Can you work these out from the model? Positions are in its coordinate system, mm. A direction names the side the tool comes from. Coordinates: 2 decimals unless noted, no trailing zeros. Order: outer loops, then holes, each group sorted by start corner. A loop starts at its lowest first (then second) coordinate and runs counter-clockwise, first axis right, second up. Notation, with made-up numbers: (-2.75, 68) -> (4.25, 68) arc R23 ccw to (4.25, 97) -> close; hole circle Ø5 at (26.25, -36.5). An arc over 180 degrees is marked (long way). Answer as CSV lines item,"result".
from build123d import *

# Parameters (mm, degrees)
SALIENTE_EXTRUIR1_DEPTH           = 10.5
CORTAR_EXTRUIR2_REACH             = 29.665
CROQUIS1_6_R                      = 1.15
CORTAR_EXTRUIR2_DIRECTION_2_REACH = 29.665
VACIADO3_T                        = -1
VACIADO3_THICKNESS_2_DEPTH        = 1
SALIENTE_EXTRUIR2_START           = 10.5
SALIENTE_EXTRUIR2_DEPTH           = 0.5
CROQUIS4_R                        = 1.15
CORTAR_EXTRUIR3_DEPTH             = 1
CROQUIS5_W                        = 6.4
CROQUIS5_H                        = 3.4
CORTAR_EXTRUIR4_DEPTH             = 0.8
CHAFL_N2_SIZE                     = 0.5
SALIENTE_EXTRUIR3_START           = -0.8
CROQUIS5_3_W                      = 6.2
CROQUIS5_3_H                      = 3.2
CROQUIS5_3_W_2                    = 5.6
CROQUIS5_3_H_2                    = 2.6
SALIENTE_EXTRUIR3_DEPTH           = 1.5
CROQUIS5_4_W                      = 5.4
CROQUIS5_4_H                      = 7.9
CORTAR_EXTRUIR5_DEPTH             = 35.965840473
SALIENTE_EXTRUIR4_START           = -0.8
CROQUIS5_6_R                      = 0.3
SALIENTE_EXTRUIR4_DEPTH           = 1.4
CROQUIS5_7_W                      = 1.3
CROQUIS5_7_H                      = 21
SALIENTE_EXTRUIR5_DEPTH           = 0.6


with BuildPart() as part:
    # Croquis1 → Saliente-Extruir1 (new, symmetric)
    with BuildSketch(Plane(origin=(0, 0, 0), x_dir=(1, 0, 0), z_dir=(0, 1, 0))):
        with BuildLine():
            Line((-9.7, 22.5), (9.7, 22.5))
            ThreePointArc((9.7, 22.5), (11.467766953, 21.767766953), (12.2, 20))
            Line((12.2, 20), (12.2, -20))
            ThreePointArc((12.2, -20), (11.467766953, -21.767766953), (9.7, -22.5))
            Line((9.7, -22.5), (-9.7, -22.5))
            ThreePointArc((-9.7, -22.5), (-11.467766953, -21.767766953), (-12.2, -20))
            Line((-12.2, -20), (-12.2, 20))
            ThreePointArc((-12.2, 20), (-11.467766953, 21.767766953), (-9.7, 22.5))
        make_face()
    extrude(amount=SALIENTE_EXTRUIR1_DEPTH, both=True)

    # Croquis1<6> → Cortar-Extruir2 (cut, up to next)
    with BuildSketch(Plane(origin=(0, 0, 0), x_dir=(1, 0, 0), z_dir=(0, 1, 0)), mode=Mode.PRIVATE) as cortar_extruir2_sk1:
        with Locations(Location((-9.93, 20.23, 0), (0, 0, 270))):
            Circle(CROQUIS1_6_R)
    cortar_extruir2_tool1 = extrude(cortar_extruir2_sk1.sketch, amount=-CORTAR_EXTRUIR2_REACH, mode=Mode.PRIVATE) & part.part
    # Croquis1<6> → Cortar-Extruir2 (cut, up to next)
    with BuildSketch(Plane(origin=(0, 0, 0), x_dir=(1, 0, 0), z_dir=(0, 1, 0)), mode=Mode.PRIVATE) as cortar_extruir2_sk2:
        with Locations(Location((9.93, 20.23, 0), (0, 0, 270))):
            Circle(CROQUIS1_6_R)
    cortar_extruir2_tool2 = extrude(cortar_extruir2_sk2.sketch, amount=-CORTAR_EXTRUIR2_REACH, mode=Mode.PRIVATE) & part.part
    # Croquis1<6> → Cortar-Extruir2 (cut, up to next)
    with BuildSketch(Plane(origin=(0, 0, 0), x_dir=(1, 0, 0), z_dir=(0, 1, 0)), mode=Mode.PRIVATE) as cortar_extruir2_sk3:
        with Locations(Location((-9.93, -20.23, 0), (0, 0, 270))):
            Circle(CROQUIS1_6_R)
    cortar_extruir2_tool3 = extrude(cortar_extruir2_sk3.sketch, amount=-CORTAR_EXTRUIR2_REACH, mode=Mode.PRIVATE) & part.part
    # Croquis1<6> → Cortar-Extruir2 (cut, up to next)
    with BuildSketch(Plane(origin=(0, 0, 0), x_dir=(1, 0, 0), z_dir=(0, 1, 0)), mode=Mode.PRIVATE) as cortar_extruir2_sk4:
        with Locations(Location((9.93, -20.23, 0), (0, 0, 270))):
            Circle(CROQUIS1_6_R)
    cortar_extruir2_tool4 = extrude(cortar_extruir2_sk4.sketch, amount=-CORTAR_EXTRUIR2_REACH, mode=Mode.PRIVATE) & part.part
    add(cortar_extruir2_tool1.solids().sort_by_distance((-9.93, 0, -20.23))[0], mode=Mode.SUBTRACT)
    add(cortar_extruir2_tool2.solids().sort_by_distance((9.93, 0, -20.23))[0], mode=Mode.SUBTRACT)
    add(cortar_extruir2_tool3.solids().sort_by_distance((-9.93, 0, 20.23))[0], mode=Mode.SUBTRACT)
    add(cortar_extruir2_tool4.solids().sort_by_distance((9.93, 0, 20.23))[0], mode=Mode.SUBTRACT)

    # Croquis1<6> → Cortar-Extruir2 direction 2 (cut, up to next)
    with BuildSketch(Plane(origin=(0, 0, 0), x_dir=(1, 0, 0), z_dir=(0, 1, 0)), mode=Mode.PRIVATE) as cortar_extruir2_direction_2_sk1:
        with Locations(Location((-9.93, 20.23, 0), (0, 0, 270))):
            Circle(CROQUIS1_6_R)
    cortar_extruir2_direction_2_tool1 = extrude(cortar_extruir2_direction_2_sk1.sketch, amount=CORTAR_EXTRUIR2_DIRECTION_2_REACH, mode=Mode.PRIVATE) & part.part
    # Croquis1<6> → Cortar-Extruir2 direction 2 (cut, up to next)
    with BuildSketch(Plane(origin=(0, 0, 0), x_dir=(1, 0, 0), z_dir=(0, 1, 0)), mode=Mode.PRIVATE) as cortar_extruir2_direction_2_sk2:
        with Locations(Location((9.93, 20.23, 0), (0, 0, 270))):
            Circle(CROQUIS1_6_R)
    cortar_extruir2_direction_2_tool2 = extrude(cortar_extruir2_direction_2_sk2.sketch, amount=CORTAR_EXTRUIR2_DIRECTION_2_REACH, mode=Mode.PRIVATE) & part.part
    # Croquis1<6> → Cortar-Extruir2 direction 2 (cut, up to next)
    with BuildSketch(Plane(origin=(0, 0, 0), x_dir=(1, 0, 0), z_dir=(0, 1, 0)), mode=Mode.PRIVATE) as cortar_extruir2_direction_2_sk3:
        with Locations(Location((-9.93, -20.23, 0), (0, 0, 270))):
            Circle(CROQUIS1_6_R)
    cortar_extruir2_direction_2_tool3 = extrude(cortar_extruir2_direction_2_sk3.sketch, amount=CORTAR_EXTRUIR2_DIRECTION_2_REACH, mode=Mode.PRIVATE) & part.part
    # Croquis1<6> → Cortar-Extruir2 direction 2 (cut, up to next)
    with BuildSketch(Plane(origin=(0, 0, 0), x_dir=(1, 0, 0), z_dir=(0, 1, 0)), mode=Mode.PRIVATE) as cortar_extruir2_direction_2_sk4:
        with Locations(Location((9.93, -20.23, 0), (0, 0, 270))):
            Circle(CROQUIS1_6_R)
    cortar_extruir2_direction_2_tool4 = extrude(cortar_extruir2_direction_2_sk4.sketch, amount=CORTAR_EXTRUIR2_DIRECTION_2_REACH, mode=Mode.PRIVATE) & part.part
    add(cortar_extruir2_direction_2_tool1.solids().sort_by_distance((-9.93, 0, -20.23))[0], mode=Mode.SUBTRACT)
    add(cortar_extruir2_direction_2_tool2.solids().sort_by_distance((9.93, 0, -20.23))[0], mode=Mode.SUBTRACT)
    add(cortar_extruir2_direction_2_tool3.solids().sort_by_distance((-9.93, 0, 20.23))[0], mode=Mode.SUBTRACT)
    add(cortar_extruir2_direction_2_tool4.solids().sort_by_distance((9.93, 0, 20.23))[0], mode=Mode.SUBTRACT)

    # Vaciado3
    vaciado3_openings = [part.faces().sort_by_distance(p)[0] for p in [
        (0, -10.5, 0),
    ]]
    offset(amount=VACIADO3_T, openings=vaciado3_openings, kind=Kind.INTERSECTION)

    # Vaciado3 thickness 2 face (on inner face of the shell) → Vaciado3 thickness 2 (add)
    with BuildSketch(Plane.ZX.offset(9.5)):
        with BuildLine():
            Line((-21.5, -8.195180125), (-21.5, 8.195180125))
            ThreePointArc((-21.5, 8.195180125), (-18.70972042, 8.40972042), (-18.495180125, 11.2))
            Line((-18.495180125, 11.2), (18.495180125, 11.2))
            ThreePointArc((18.495180125, 11.2), (18.70972042, 8.40972042), (21.5, 8.195180125))
            Line((21.5, 8.195180125), (21.5, -8.195180125))
            ThreePointArc((21.5, -8.195180125), (18.70972042, -8.40972042), (18.495180125, -11.2))
            Line((18.495180125, -11.2), (-18.495180125, -11.2))
            ThreePointArc((-18.495180125, -11.2), (-18.70972042, -8.40972042), (-21.5, -8.195180125))
        make_face()
    extrude(amount=-VACIADO3_THICKNESS_2_DEPTH)

    # Croquis1<4> → Saliente-Extruir2 (add)
    with BuildSketch(Plane(origin=(0, 0, 0), x_dir=(1, 0, 0), z_dir=(0, 1, 0)).offset(SALIENTE_EXTRUIR2_START)):
        with BuildLine():
            ThreePointArc((9.7, 22), (11.114213562, 21.414213562), (11.7, 20))
            Line((11.7, 20), (11.7, -20))
            ThreePointArc((11.7, -20), (11.114213562, -21.414213562), (9.7, -22))
            Line((9.7, -22), (-9.7, -22))
            ThreePointArc((-9.7, -22), (-11.114213562, -21.414213562), (-11.7, -20))
            Line((-11.7, -20), (-11.7, 20))
            ThreePointArc((-11.7, 20), (-11.114213562, 21.414213562), (-9.7, 22))
            Line((-9.7, 22), (9.7, 22))
        make_face()
        with BuildLine():
            ThreePointArc((-9.7, 21.5), (-10.760660172, 21.060660172), (-11.2, 20))
            Line((-11.2, 20), (-11.2, -20))
            ThreePointArc((-11.2, -20), (-10.760660172, -21.060660172), (-9.7, -21.5))
            Line((-9.7, -21.5), (9.7, -21.5))
            ThreePointArc((9.7, -21.5), (10.760660172, -21.060660172), (11.2, -20))
            Line((11.2, -20), (11.2, 20))
            ThreePointArc((11.2, 20), (10.760660172, 21.060660172), (9.7, 21.5))
            Line((9.7, 21.5), (-9.7, 21.5))
        make_face(mode=Mode.SUBTRACT)
    saliente_extruir2 = extrude(amount=SALIENTE_EXTRUIR2_DEPTH)

    # Simetría3: Saliente-Extruir2 across plane
    add(saliente_extruir2.mirror(Plane.ZX))

    # Croquis4 → Cortar-Extruir3 (cut)
    with BuildSketch(Plane(origin=(0, 10.5, 0), x_dir=(1, 0, 0), z_dir=(0, 1, 0))):
        with BuildLine():
            Line((11.2, -20), (11.2, 20))
            ThreePointArc((11.2, 20), (10.760660172, 21.060660172), (9.7, 21.5))
            Line((9.7, 21.5), (-9.7, 21.5))
            ThreePointArc((-9.7, 21.5), (-10.760660172, 21.060660172), (-11.2, 20))
            Line((-11.2, 20), (-11.2, -20))
            ThreePointArc((-11.2, -20), (-10.760660172, -21.060660172), (-9.7, -21.5))
            Line((-9.7, -21.5), (9.7, -21.5))
            ThreePointArc((9.7, -21.5), (10.760660172, -21.060660172), (11.2, -20))
        make_face()
        with Locations(Location((-9.93, -20.23, 0), (0, 0, 270))):
            Circle(CROQUIS4_R, mode=Mode.SUBTRACT)
        with Locations(Location((9.93, -20.23, 0), (0, 0, 270))):
            Circle(CROQUIS4_R, mode=Mode.SUBTRACT)
        with Locations(Location((-9.93, 20.23, 0), (0, 0, 270))):
            Circle(CROQUIS4_R, mode=Mode.SUBTRACT)
        with Locations(Location((9.93, 20.23, 0), (0, 0, 270))):
            Circle(CROQUIS4_R, mode=Mode.SUBTRACT)
    extrude(amount=-CORTAR_EXTRUIR3_DEPTH, mode=Mode.SUBTRACT)

    # Croquis5 → Cortar-Extruir4 (cut)
    with BuildSketch(Plane.ZY.offset(12.2)):
        with Locations((-4.9, -3)):
            Rectangle(CROQUIS5_W, CROQUIS5_H)
    extrude(amount=-CORTAR_EXTRUIR4_DEPTH, mode=Mode.SUBTRACT)

    # Chaflán2
    chafl_n2_edges = [part.edges().sort_by_distance(p)[0] for p in [
        (-12.2, -4.7, -4.9),
        (-12.2, -3, -8.1),
        (-12.2, -3, -1.7),
        (-12.2, -1.3, -4.9),
    ]]
    chamfer(chafl_n2_edges, length=CHAFL_N2_SIZE)

    # Croquis5<4> → Cortar-Extruir5 (cut, through all)
    with BuildSketch(Plane.ZY.offset(12.2)):
        with Locations((12.135332852, 1.782001246)):
            Rectangle(CROQUIS5_4_W, CROQUIS5_4_H)
    extrude(amount=-CORTAR_EXTRUIR5_DEPTH, mode=Mode.SUBTRACT)


with BuildPart() as body_2:
    # Croquis5<3> → Saliente-Extruir3 (new body)
    with BuildSketch(Plane.ZY.offset(12.2).offset(SALIENTE_EXTRUIR3_START)):
        with Locations((-4.9, -3)):
            Rectangle(CROQUIS5_3_W, CROQUIS5_3_H)
        with Locations((-4.9, -3)):
            Rectangle(CROQUIS5_3_W_2, CROQUIS5_3_H_2, mode=Mode.SUBTRACT)
    extrude(amount=SALIENTE_EXTRUIR3_DEPTH)


    add(part.part)  # Saliente-Extruir4 merges part
    # Croquis5<6> → Saliente-Extruir4 (add)
    with BuildSketch(Plane.ZY.offset(12.2).offset(SALIENTE_EXTRUIR4_START)):
        with Locations(Location((-6.9, -3, 0), (0, 0, 180))):
            Circle(CROQUIS5_6_R)
        with Locations(Location((-4.9, -3, 0), (0, 0, 180))):
            Circle(CROQUIS5_6_R)
        with Locations(Location((-2.9, -3, 0), (0, 0, 180))):
            Circle(CROQUIS5_6_R)
    extrude(amount=SALIENTE_EXTRUIR4_DEPTH)

    # Croquis5<7> → Saliente-Extruir5 (add)
    with BuildSketch(Plane.ZY.offset(12.2)):
        with Locations((19.35, 0)):
            Rectangle(CROQUIS5_7_W, CROQUIS5_7_H)
    saliente_extruir5 = extrude(amount=SALIENTE_EXTRUIR5_DEPTH)

    # Simetría4: Saliente-Extruir5 across plane
    add(saliente_extruir5.mirror(Plane(origin=(0, 0, 0), x_dir=(0, 0, 1), z_dir=(1, 0, 0))))


solid = body_2.part
Q1. Which directions (+Z, -Z, +X, -X, +Y, -Y) give clear straight access to the entire face, cutting with the end or side of a thin tool? Please do faces 5 (the flat face through (-11.2, -1, 0)), 6 (the flat face through (-12, 2, 14.835)), 7 (the cylindrical face through (-11.13, -10.75, -21.4)), 8 (the flat face through (-12, -1.7, -5)).
Solution:
face 5,"-Y"
face 6,"+X, -X"
face 7,"-Z, -X, -Y"
face 8,"-X"
Q2. Imagine slicing it at B-B (z = -14). List the corners of the cut face in (x, y) for me.
Solution:
outline,"(-12.2, -10.5) -> (-11.7, -10.5) -> (-11.7, -11) -> (-11.2, -11) -> (-11.2, 8.5) -> (11.2, 8.5) -> (11.2, -11) -> (11.7, -11) -> (11.7, -10.5) -> (12.2, -10.5) -> (12.2, 10.5) -> (11.7, 10.5) -> (11.7, 11) -> (11.2, 11) -> (11.2, 9.5) -> (-11.2, 9.5) -> (-11.2, 11) -> (-11.7, 11) -> (-11.7, 10.5) -> (-12.2, 10.5) -> close"
Q3. Imagine slicing it at A-A (y = 3). Give the number of separate pieces and of enclosed holes in the cut face, and give its area (3 significant figures).
Solution:
separate pieces,"2"
enclosed holes,"4"
area,"145 mm2"
Q4. Imagine slicing it at D-D (y = 6.5). List the corners of the cut face in (x, z) for me.
Solution:
outline,"(-12.8, 18.7) -> (-12.2, 18.7) -> (-12.2, -20) arc R2.5 ccw to (-9.7, -22.5) -> (9.7, -22.5) arc R2.5 ccw to (12.2, -20) -> (12.2, 18.7) -> (12.8, 18.7) -> (12.8, 20) -> (12.2, 20) arc R2.5 ccw to (9.7, 22.5) -> (-9.7, 22.5) arc R2.5 ccw to (-12.2, 20) -> (-12.8, 20) -> close; hole (-11.2, -18.5) arc R2.15 cw to (-8.2, -21.5) -> (8.2, -21.5) arc R2.15 cw to (11.2, -18.5) -> (11.2, 18.5) arc R2.15 cw to (8.2, 21.5) -> (-8.2, 21.5) arc R2.15 cw to (-11.2, 18.5) -> close; hole circle Ø2.3 at (-9.93, -20.23); hole circle Ø2.3 at (-9.93, 20.23); hole circle Ø2.3 at (9.93, -20.23); hole circle Ø2.3 at (9.93, 20.23)"
Q5. If I drill on line 1 (X direction, y = 4.25, z = -20.23); line 2 (X direction, y = -7.25, z = -1); line 3 (Z direction, x = -5.25, y = 3.5), over which ranges is the centre line in solid material (lowest first)?
Solution:
line 1,"-12.19 to -11.08, -8.78 to -7.78, 7.78 to 8.78, 11.08 to 12.19"
line 2,"-12.2 to -11.2, 11.2 to 12.2"
line 3,"-22.5 to -21.5, 21.5 to 22.5"
Q6. For P1, Ø1.2, axis at x = -12.5, y = -3, coming from the -Z side; P2, Ø3, axis at x = 6.5, z = 6, coming from the -Y side; P3, Ø3, axis at y = 4.5, z = -1, coming from the -X side, each with a flat end and sliding along its axis, tell me the tip position at first contact or that it passes through.
Solution:
P1,"z = -21.19"
P2,"y = 8.5"
P3,"x = -12.2"
Q7. We'd pull the mould along X, two halves only. Please class faces 1 (the cylindrical face through (11.1, -10.75, -21.43)), 2 (the cylindrical face through (10.77, -10.75, -21.05)), 3 (the flat face through (-12, 5.732, 12)), 4 (the cylindrical face through (-11.487, 0.147, -21.748)): pulls with the +X half, pulls with the -X half, needs draft (parallel to the pull), parting line crosses it, or undercut.
Solution:
face 1,"pulls with the +X half"
face 2,"undercut"
face 3,"needs draft"
face 4,"pulls with the -X half"
Q8. Imagine slicing it at C-C (x = -3.5). List the corners of the cut face in (y, z) for me, and give its area (3 significant figures).
Solution:
outline,"(-11, -22) -> (-10.5, -22) -> (-10.5, -22.5) -> (10.5, -22.5) -> (10.5, -22) -> (11, -22) -> (11, -21.5) -> (9.5, -21.5) -> (9.5, 21.5) -> (11, 21.5) -> (11, 22) -> (10.5, 22) -> (10.5, 22.5) -> (-10.5, 22.5) -> (-10.5, 22) -> (-11, 22) -> (-11, 21.5) -> (8.5, 21.5) -> (8.5, -21.5) -> (-11, -21.5) -> close"
area,"86.0 mm2"
